```python
from build123d import *

# Parameters (mm, degrees)
F1_R     = 25.4
F1_R_2   = 20.32
F2_DEPTH = 7.62
F3_R     = 3.81
F0_R     = 3.80999


# Not quite as in the source:
# - a fillet or chamfer is up to 0.001 mm smaller than in the source, because OpenCascade refuses the exact size


with BuildPart() as f2:
    # F1 (on Top) → F2 (new body)
    with BuildSketch(Plane.XY):
        Circle(F1_R)
        Circle(F1_R_2, mode=Mode.SUBTRACT)
    extrude(amount=F2_DEPTH)

    # F3
    f3_edges = [f2.edges().sort_by_distance(p)[0] for p in [
        (-25.4, 0, 0),
    ]]
    fillet(f3_edges, radius=F3_R)

    # F0 (radius 3.81 in the source; OpenCascade refuses exactly that, so slightly less here)
    f0_edges = [f2.edges().sort_by_distance(p)[0] for p in [
        (-25.4, 0, 7.62),
    ]]
    fillet(f0_edges, radius=F0_R)


solid = f2.part
```
Source: CAD feature listing. Evaluate the final solid. Frame: model axes, mm. Give positions to 0.01 mm unless a question says otherwise; leave off trailing zeros. Write each loop counter-clockwise with the first axis right and the second up, starting at its lowest first coordinate (ties: lowest second). Pieces come first, ordered by that corner, then holes.
1. First-contact query: pin 1 (2 mm diameter, centred on y = -7.5, z = 1.5, fed in from -X); pin 2 (4 mm diameter, centred on x = 16.5, y = -1.5, fed in from +Z); pin 3 (3 mm diameter, centred on y = -8.5, z = 2.5, fed in from +X). Flat tips, straight axial feed; report the tip coordinate or a pass-through.
2. Section query D-D (z = 6.5). Return the cut outline in (x, y), then the cut area to 3 significant figures.
3. Section query C-C (z = 2.25). Return the cut outline in (x, y).
4. Material intervals for line 1 along X through (y, z) = (16, 1.5); line 2 along X through (y, z) = (6.5, 5.25); line 3 along Y through (x, z) = (14.5, 2.5), sorted ascending.
5. Pull-direction query (Y, two-part tool) for faces 1 (the face through (13, -16, 7.62)), 2 (the face through (-2.645, 20.147, 3.757)); classes: +Y half, -Y half, draft (parallel to the pull), parting line (faces both ways), or undercut.
Output values:
1. pin 1: stops at x = -24.12
1. pin 2: passes through
1. pin 3: stops at x = 24.31
2. outline: circle Ø48.58 at (0, 0); hole circle Ø40.64 at (0, 0)
2. area: 556 mm2
3. outline: circle Ø50.13 at (0, 0); hole circle Ø40.64 at (0, 0)
4. line 1: x = -18.71 to -12.53, 12.53 to 18.71
4. line 2: x = -24.26 to -19.25, 19.25 to 24.26
4. line 3: y = -20.57 to -14.24, 14.24 to 20.57
5. face 1: draft
5. face 2: undercut
